Geometry: final body of the model. Coordinates: model frame, mm. A direction names the side the tool comes from. Give positions to 0.01 mm unless a question says otherwise; leave off trailing zeros. Order: outer loops, then holes, each group sorted by start corner. A loop starts at its lowest first (then second) coordinate and runs counter-clockwise, first axis right, second up. Notation, with made-up numbers: (35, 80.25) -> (60, 80.25) arc R21 ccw to (60, 112.25) -> close; hole circle Ø5 at (67.5, 15). An arc over 180 degrees is marked (long way). Answer in a Markdown table with one row per item. Add a question column.
Q1. Pull-direction query (X, two-part tool) for faces 1 (the face through (104, 86, 0)), 2 (the face through (-104, 86, 0)), 3 (the face through (55, 15, 0)), 4 (the face through (-1, 86, 10)); classes: +X half, -X half, draft (parallel to the pull), parting line (faces both ways), or undercut.
Q2. Set-up query: faces 5 (the face through (87, 163, 0)), 6 (the face through (-1, 0, 0)), 7 (the face through (-55, 15, 0)). Return all of +Z, -Z, +X, -X, +Y, -Y with unobstructed straight access to the full face (end or side cutting, diameter ignored); none if empty.
Q3. Cut plane A-A on x = -87.5. Return the cut outline in (y, z), and give its area (3 significant figures).
Q4. Line query: line 1 along X through (y, z) = (8, 0); line 2 along X through (y, z) = (170.25, 0); line 3 along Z through (x, y) = (87, 170). Output: solid intervals per line, ascending. Write a range as from..to.
Q5. Contact query for flat-ended pins moving along their axis: P1, Ø7, axis at x = 0, z = 0, coming from the +Y side; P2, Ø4, axis at x = -54.5, z = 1.5, coming from the -Y side; P3, Ø6.5, axis at x = 88.5, z = -0.5, coming from the +Y side. Output: stop coordinate, or through.
from build123d import *

# Parameters (mm, degrees)
SKETCH1_W           = 208
SKETCH1_H           = 20
BOSS_EXTRUDE1_DEPTH = 175
SKETCH2_R           = 4
CUT_EXTRUDE1_DEPTH  = 12
SKETCH3_R           = 4
CUT_EXTRUDE2_DEPTH  = 15
CHAMFER1_SIZE       = 0.5


with BuildPart() as part:
    # Sketch1 → Boss-Extrude1 (new body)
    with BuildSketch(Plane(origin=(0, 0, -58), x_dir=(1, 0, 0), z_dir=(0, 1, 0))):
        with Locations((0, -58)):
            Rectangle(SKETCH1_W, SKETCH1_H)
    extrude(amount=BOSS_EXTRUDE1_DEPTH)

    # Sketch2 → Cut-Extrude1 (cut)
    with BuildSketch(Plane(origin=(0, 175, 0), x_dir=(1, 0, 0), z_dir=(0, 1, 0))):
        with Locations(Location((0, 0, 0), (0, 0, 270))):
            Circle(SKETCH2_R)
        with Locations(Location((-87.5, 0, 0), (0, 0, 270))):
            Circle(SKETCH2_R)
        with Locations(Location((87.5, 0, 0), (0, 0, 90))):
            Circle(SKETCH2_R)
    extrude(amount=-CUT_EXTRUDE1_DEPTH, mode=Mode.SUBTRACT)

    # Sketch3 → Cut-Extrude2 (cut)
    with BuildSketch(Plane.XZ):
        with Locations(Location((-55, 0, 0), (0, 0, 270))):
            Circle(SKETCH3_R)
        with Locations(Location((55, 0, 0), (0, 0, 90))):
            Circle(SKETCH3_R)
    extrude(amount=-CUT_EXTRUDE2_DEPTH, mode=Mode.SUBTRACT)

    # Chamfer1
    chamfer1_edges = [part.edges().sort_by_distance(p)[0] for p in [
        (87.5, 175, 4),
        (-87.5, 175, -4),
        (0, 175, -4),
        (-55, 0, 4),
        (55, 0, -4),
    ]]
    chamfer(chamfer1_edges, length=CHAMFER1_SIZE)


solid = part.part
Completed:
| question | item | result |
|---|---|---|
| 1 | face 1 | +X half |
| 1 | face 2 | -X half |
| 1 | face 3 | undercut |
| 1 | face 4 | draft |
| 2 | face 5 | +Y |
| 2 | face 6 | +Z, -Z, +X, -X, -Y |
| 2 | face 7 | -Y |
| 3 | outline | (0, -10) -> (175, -10) -> (175, -4.5) -> (174.5, -4) -> (163, -4) -> (163, 4) -> (174.5, 4) -> (175, 4.5) -> (175, 10) -> (0, 10) -> close |
| 3 | area | 3,400 mm² |
| 4 | line 1 | x = -104..-59, -51..51, 59..104 |
| 4 | line 2 | x = -104..-91.5, -83.5..-4, 4..83.5, 91.5..104 |
| 4 | line 3 | z = -10..-3.97, 3.97..10 |
| 5 | P1 | stops at y = 163 |
| 5 | P2 | stops at y = 15 |
| 5 | P3 | stops at y = 174.87 |
